Can you work these out from the model? Positions are in its coordinate system, mm. Round coordinates to 2 decimals unless told otherwise and drop trailing zeros. Loops run counter-clockwise (first coordinate to the right, second up) from the corner with the lowest first, then second, coordinate; pieces in that order, holes last. Notation, with made-up numbers: M -16,31.5 L 31,31.5 A35 ccw 31,64.5 Z; hole C 75.5,60.25 d9. An arc over 180 degrees is marked long. Return JSON: item names as keys, results as strings.
```python
from build123d import *

# Parameters (mm, degrees)
F0_W     = 254
F0_H     = 76.2
F1_DEPTH = 6.35
F2_R     = 9.525
F3_DEPTH = 25.4
F4_R     = 3.175


with BuildPart() as f1:
    # F0 (on Top) → F1 (new body)
    with BuildSketch(Plane.XY):
        with Locations((127, -38.1)):
            Rectangle(F0_W, F0_H)
    extrude(amount=-F1_DEPTH)

    # F2 (on face) → F3 (cut)
    with BuildSketch(Plane.XY):
        with Locations((63.5, -50.8)):
            Circle(F2_R)
        with Locations((190.5, -50.8)):
            Circle(F2_R)
    extrude(amount=-F3_DEPTH, mode=Mode.SUBTRACT)

    # F4
    f4_edges = [f1.edges().sort_by_distance(p)[0] for p in [
        (254, -76.2, -3.175),
        (254, 0, -3.175),
        (0, -76.2, -3.175),
        (0, 0, -3.175),
    ]]
    fillet(f4_edges, radius=F4_R)


solid = f1.part
```
Q1. If I drill on line 1 along Y through (x, z) = (63, -3); line 2 along X through (y, z) = (-55.5, -2); line 3 along Y through (x, z) = (182.5, -5.5), over which ranges is the centre line in solid material (lowest first)?
Results:
{"line 1": "y = -76.2 to -60.31, -41.29 to 0", "line 2": "x = 0 to 55.22, 71.78 to 182.22, 198.78 to 254", "line 3": "y = -76.2 to -55.97, -45.63 to 0"}
Q2. I'm going to push a flat-ended pin straight in: pin 1 Ø22 at (x, y) = (190.5, -50.8) entering from -Z. Where does the tip first touch, or does it pass through?
Results:
{"pin 1": "stops at z = -6.35"}
Q3. Suppose I cut it at D-D, the plane x = 184.5. Please give me the cut outline in (y, z).
Results:
{"outline": "M -76.2,-6.35 L -58.2,-6.35 L -58.2,0 L -76.2,0 Z; M -43.4,-6.35 L 0,-6.35 L 0,0 L -43.4,0 Z"}
Q4. Suppose I cut it at B-B, the plane y = -50.8. Please give me the cut outline in (x, z) (3 decimals).
Results:
{"outline": "M 0,-6.35 L 53.975,-6.35 L 53.975,0 L 0,0 Z; M 73.025,-6.35 L 180.975,-6.35 L 180.975,0 L 73.025,0 Z; M 200.025,-6.35 L 254,-6.35 L 254,0 L 200.025,0 Z"}
Q5. Suppose I cut it at C-C, the plane z = -4. Please give me the cut outline in (x, y) (3 decimals).
Results:
{"outline": "M 0,-73.025 A3.175 ccw 3.175,-76.2 L 250.825,-76.2 A3.175 ccw 254,-73.025 L 254,-3.175 A3.175 ccw 250.825,0 L 3.175,0 A3.175 ccw 0,-3.175 Z; hole C 63.5,-50.8 d19.05; hole C 190.5,-50.8 d19.05"}
Q6. Suppose I cut it at A-A, the plane x = 63.5. Please give me the cut outline in (y, z) (3 decimals), plus the area to 3 significant figures.
Results:
{"outline": "M -76.2,-6.35 L -60.325,-6.35 L -60.325,0 L -76.2,0 Z; M -41.275,-6.35 L 0,-6.35 L 0,0 L -41.275,0 Z", "area": "363 mm2"}
Q7. Thinking about a two-plate mould opening in X: for faces 1 (the flat face through (254, -39, -3)), 2 (the cylindrical face through (180.984, -50.381, -3.131)), 3 (the flat face through (125, -38, -6.35)), which applies, pulls with the +X half, pulls with the -X half, needs draft (parallel to the pull), parting line crosses it, or undercut?
Results:
{"face 1": "pulls with the +X half", "face 2": "undercut", "face 3": "needs draft"}
